Read the model definition and answer for the solid it produces. Units are mm, in the model's axes. A direction names the side the tool comes from. Coordinates: 2 decimals unless noted, no trailing zeros. Write each loop counter-clockwise with the first axis right and the second up, starting at its lowest first coordinate (ties: lowest second). Pieces come first, ordered by that corner, then holes. Notation, with made-up numbers: (-8.75, 82.5) -> (22.25, 82.5) arc R36 cw to (22.25, 121.5) -> close; hole circle Ø3 at (-4, 47). An arc over 180 degrees is marked (long way). Return JSON: item names as keys, results as strings.
from build123d import *

# Parameters (mm, degrees)
F0_W         = 96
F0_H         = 96
F1_DEPTH     = 103
F2_R         = 16.5
F3_DEPTH     = 100
F4_R         = 46.5
F5_DEPTH     = 80
F6_T1_DEPTH  = 106
F6_T3_DEPTH  = 106
F7_T1_DEPTH  = 110.4999999999
F7_T4_ANGLE  = 90
F7_T6_ANGLE  = 90
F7_T8_ANGLE  = 90
F7_T10_ANGLE = 90
F9_SIZE      = 2
F8_W         = 14.3129900098
F8_H         = 43.2826243341
F12_R        = 5
F13_W        = 11.0455658287
F13_H        = 45.8308011293


# Not quite as in the source:
# - a fillet or chamfer that OpenCascade refuses, or shapes differently, is made with other operations: its cross-section is extruded or revolved along the edge and cut away or added


with BuildPart() as f1:
    # F0 (on Top) → F1 (new body)
    with BuildSketch(Plane.XY):
        Rectangle(F0_W, F0_H)
    extrude(amount=F1_DEPTH)

    # F2 (on face) → F3 (cut)
    with BuildSketch(Plane.XY.offset(103)):
        Circle(F2_R)
    extrude(amount=-F3_DEPTH, mode=Mode.SUBTRACT)

    # F4 (on face) → F5 (cut)
    with BuildSketch(Plane.XY.offset(103)):
        Circle(F4_R)
    extrude(amount=-F5_DEPTH, mode=Mode.SUBTRACT)

    # F6: fillet of radius 2 on 4 edges, made by hand

    # F6_s2 → F6_t1 (cut)
    with BuildSketch(Plane.YZ.offset(-53)):
        with BuildLine():
            ThreePointArc((48, 101), (47.4142135624, 102.4142135624), (46, 103))
            Line((46, 103), (48, 103))
            Line((48, 103), (48, 101))
        make_face()
        with BuildLine():
            ThreePointArc((-48, 101), (-47.4142135624, 102.4142135624), (-46, 103))
            Line((-46, 103), (-48, 103))
            Line((-48, 103), (-48, 101))
        make_face()
    extrude(amount=F6_T1_DEPTH, mode=Mode.SUBTRACT)

    # F6_s4 → F6_t3 (cut)
    with BuildSketch(Plane.XZ.offset(-53)):
        with BuildLine():
            ThreePointArc((48, 101), (47.4142135624, 102.4142135624), (46, 103))
            Line((46, 103), (48, 103))
            Line((48, 103), (48, 101))
        make_face()
        with BuildLine():
            ThreePointArc((-46, 103), (-47.4142135624, 102.4142135624), (-48, 101))
            Line((-48, 101), (-48, 103))
            Line((-48, 103), (-46, 103))
        make_face()
    extrude(amount=F6_T3_DEPTH, mode=Mode.SUBTRACT)

    # F7: fillet of radius 3 on 4 edges, made by hand

    # F7_s2 → F7_t1 (cut)
    with BuildSketch(Plane.XY.offset(-7.5)):
        with BuildLine():
            ThreePointArc((48, -45), (47.1213203436, -47.1213203436), (45, -48))
            Line((45, -48), (48, -48))
            Line((48, -48), (48, -45))
        make_face()
        with BuildLine():
            ThreePointArc((-45, -48), (-47.1213203436, -47.1213203436), (-48, -45))
            Line((-48, -45), (-48, -48))
            Line((-48, -48), (-45, -48))
        make_face()
        with BuildLine():
            ThreePointArc((-45, 48), (-47.1213203436, 47.1213203436), (-48, 45))
            Line((-48, 45), (-48, 48))
            Line((-48, 48), (-45, 48))
        make_face()
        with BuildLine():
            ThreePointArc((48, 45), (47.1213203436, 47.1213203436), (45, 48))
            Line((45, 48), (48, 48))
            Line((48, 48), (48, 45))
        make_face()
    extrude(amount=F7_T1_DEPTH, mode=Mode.SUBTRACT)

    # F7_s3 → F7_t4 (revolve, cut)
    with BuildSketch(Plane.XZ.offset(-45)):
        with BuildLine():
            ThreePointArc((46.0000000001, 103), (47.4142135624, 102.4142135624), (48, 101.0000000001))
            Line((48, 101.0000000001), (48, 103))
            Line((48, 103), (46.0000000001, 103))
        make_face()
    revolve(axis=Axis((45, 45, 103), (0, 0, 1)), revolution_arc=F7_T4_ANGLE, mode=Mode.SUBTRACT)

    # F7_s5 → F7_t6 (revolve, cut)
    with BuildSketch(Plane.YZ.offset(-45)):
        with BuildLine():
            ThreePointArc((46.0000000001, 103), (47.4142135624, 102.4142135624), (48, 101.0000000001))
            Line((48, 101.0000000001), (48, 103))
            Line((48, 103), (46.0000000001, 103))
        make_face()
    revolve(axis=Axis((-45, 45, 103), (0, 0, 1)), revolution_arc=F7_T6_ANGLE, mode=Mode.SUBTRACT)

    # F7_s7 → F7_t8 (revolve, cut)
    with BuildSketch(Plane.XZ.offset(45)):
        with BuildLine():
            ThreePointArc((-46.0000000001, 103), (-47.4142135624, 102.4142135624), (-48, 101.0000000001))
            Line((-48, 101.0000000001), (-48, 103))
            Line((-48, 103), (-46.0000000001, 103))
        make_face()
    revolve(axis=Axis((-45, -45, 103), (0, 0, 1)), revolution_arc=F7_T8_ANGLE, mode=Mode.SUBTRACT)

    # F7_s9 → F7_t10 (revolve, cut)
    with BuildSketch(Plane.YZ.offset(45)):
        with BuildLine():
            ThreePointArc((-46.0000000001, 103), (-47.4142135624, 102.4142135624), (-48, 101.0000000001))
            Line((-48, 101.0000000001), (-48, 103))
            Line((-48, 103), (-46.0000000001, 103))
        make_face()
    revolve(axis=Axis((45, -45, 103), (0, 0, 1)), revolution_arc=F7_T10_ANGLE, mode=Mode.SUBTRACT)

    # F9
    f9_edges = [f1.edges().sort_by_distance(p)[0] for p in [
        (-16.5, 0, 23),
    ]]
    chamfer(f9_edges, length=F9_SIZE)

    # F11: sweep along a path in F10
    with BuildLine(Plane.XY.offset(23)) as f11_path:
        Line((27.1213203436, -47.9204392359), (48.4205447137, -27.1213203436))
    # F8 (on face) → F11 (sweep, cut)
    with BuildSketch(Plane.XZ.offset(48)):
        with Locations((32.499153167, 69.7716791183)):
            Rectangle(F8_W, F8_H)
    sweep(path=f11_path.line, mode=Mode.SUBTRACT)

    # F12
    f12_edges = [f1.edges().sort_by_distance(p)[0] for p in [
        (-46.5, 0, 23),
    ]]
    fillet(f12_edges, radius=F12_R)

    # F13 (on face) → F14 (revolve, cut)
    with BuildSketch(Plane(origin=(-48, 0, 0), x_dir=(0, -1, 0), z_dir=(-1, 0, 0))):
        with Locations((-33.7943071499, 70.3311860561)):
            Rectangle(F13_W, F13_H)
    revolve(axis=Axis((-45, 48, 50.5), (0, 0, -1)), mode=Mode.SUBTRACT)


solid = f1.part
1. Flat-ended cylindrical pins translate along their axes: pin 1 Ø1.5 at (x, z) = (47.5, 79) entering from -Y; pin 2 Ø25 at (x, y) = (19.5, -9.5) entering from +Z. Find the tip coordinate at first contact, or state that the pin passes through.
Taken from the geometry:
{"pin 1": "stops at y = -47.44", "pin 2": "stops at z = 23"}
2. The part is cut by section C-C (x = 0). Determine the outline of the cut face in (y, z).
Taken from the geometry:
{"outline": "(-48, 0) -> (48, 0) -> (48, 101) arc R2 ccw to (46.5, 102.94) -> (46.5, 28) arc R5 cw to (41.5, 23) -> (18.5, 23) -> (16.5, 21) -> (16.5, 3) -> (-16.5, 3) -> (-16.5, 21) -> (-18.5, 23) -> (-41.5, 23) arc R5 cw to (-46.5, 28) -> (-46.5, 102.94) arc R2 ccw to (-48, 101) -> close"}
3. The part is cut by section A-A (z = 34). Determine the outline of the cut face in (x, y), then the cut area to 3 significant figures.
Taken from the geometry:
{"outline": "(-48, -45) arc R3 ccw to (-45, -48) -> (45, -48) arc R3 ccw to (48, -45) -> (48, 45) arc R3 ccw to (45, 48) -> (-45, 48) arc R3 ccw to (-48, 45) -> close; hole circle Ø93 at (0, 0)", "area": "2,420 mm2"}
4. Consider L1, parallel to Y at x = 0, z = 9; L2, parallel to Y at x = 0, z = 46; L3, parallel to X at y = -21, z = 84. Determine where each line is inside the solid, lowest interval first.
Taken from the geometry:
{"L1": "y = -48 to -16.5, 16.5 to 48", "L2": "y = -48 to -46.5, 46.5 to 48", "L3": "x = -48 to -41.49, 41.49 to 48"}
5. The part is cut by section B-B (z = 67.5). Determine the outline of the cut face in (x, y), then the cut area to 3 significant figures.
Taken from the geometry:
{"outline": "(-48, -45) arc R3 ccw to (-45, -48) -> (25.34, -48) -> (46.64, -27.2) -> (48, -27.2) -> (48, 45) arc R3 ccw to (45, 48) -> (-25.04, 48) arc R19.96 cw to (-28.55, 36.7) arc R46.5 cw (long way) to (-34.79, 30.86) arc R19.96 cw to (-48, 28.27) -> close; (-48, 39.32) arc R9.19 ccw to (-35.81, 48) -> (-45, 48) arc R3 ccw to (-48, 45) -> close; (39.66, -48) -> (45, -48) arc R3 ccw to (48, -45) -> (48, -39.85) -> close", "area": "1,920 mm2"}
6. A tool of negligible diameter and unlimited length cuts with its end or side. For faces 4 (the face through (21.46, -41.25, 66.03)), 5 (the face through (-25.916, 42.166, 70.652)), 6 (the face through (39, -40, 91.413)), from which of +Z, -Z, +X, -X, +Y, -Y can it reach the whole face along a straight path? Write none if from no direction.
Taken from the geometry:
{"face 4": "+Z", "face 5": "+Y", "face 6": "none"}
7. For a pull along Z with two mould halves and no side action, classify faces 1 (the face through (18, -9, 23)), 2 (the face through (-1, 1, 0)), 3 (the face through (39, -40, 48.13)) as +Z half, -Z half, draft (parallel to the pull), parting line (faces both ways), or undercut.
Taken from the geometry:
{"face 1": "+Z half", "face 2": "-Z half", "face 3": "undercut"}
